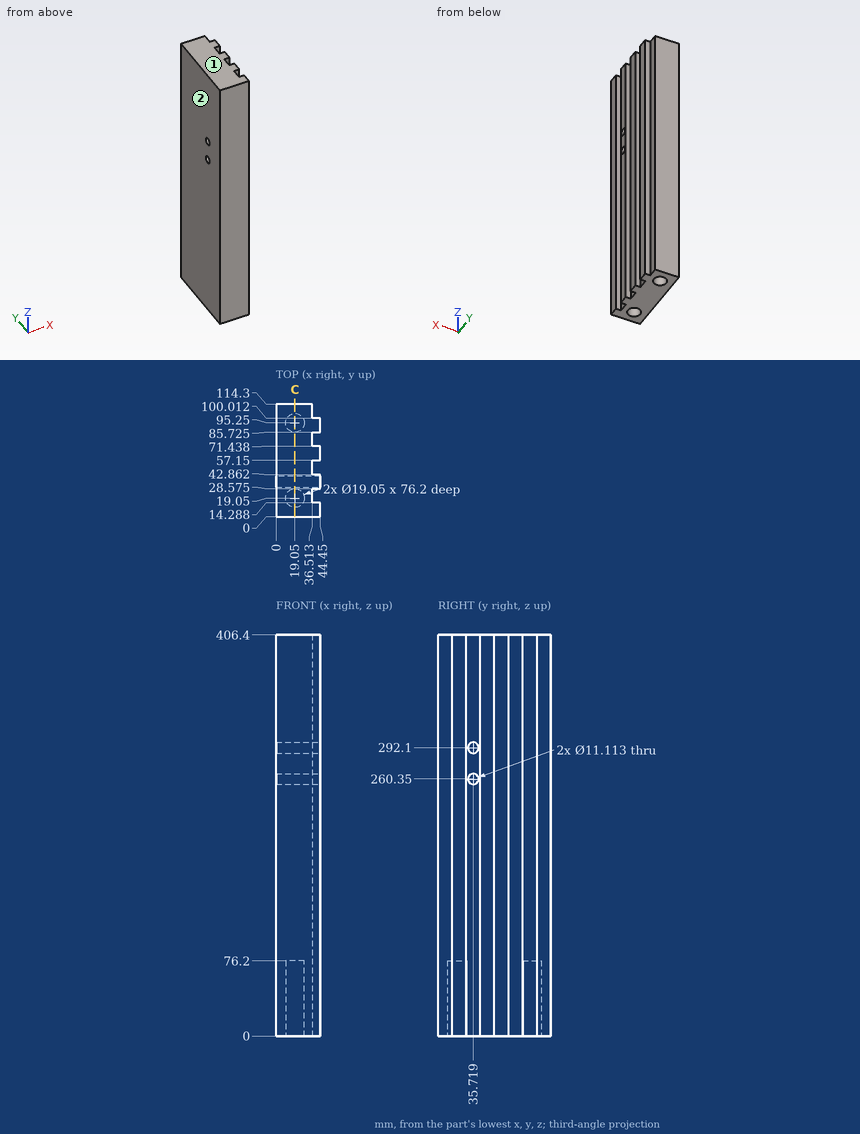
Here's the drawing with two shaded views (mm, measured from the low corner). I have some questions. Round coordinates to 2 decimals unless told otherwise and drop trailing zeros.
Item 1: If we mould it in two halves opening along X, with no side actions, what happens to the marked faces 1 and 2? For each: +X half, -X half, draft (parallel to the pull), parting line (faces both ways), or undercut.
Item 2: Suppose I cut it at C-C, the plane x = 19.05. State how many separate pieces and enclosed holes the cut face has, then the cut area to 3 significant figures.
Item 3: Will these pins go through, and if not, where does the flat tip stop? pin 1 Ø5.5 at (x, y) = (18, 97.5) entering from -Z; pin 2 Ø6 at (y, z) = (43.5, 94.5) entering from -X; pin 3 Ø7 at (y, z) = (18, 230.5) entering from +X; pin 4 Ø2.5 at (x, z) = (39.5, 171) entering from +Y.
Item 4: Please list where these lines run through material, in increasing order: L1, parallel to Y at x = 19.05, z = 42 (1 decimal); L2, parallel to X at y = 19, z = 16 (1 decimal); L3, parallel to Y at x = 16, z = 292 (1 decimal).
Reported:
1. face 1: draft
1. face 2: -X half
2. separate pieces: 1
2. enclosed holes: 2
2. area: 43,400 mm2
3. pin 1: stops at z = 76.2
3. pin 2: stops at x = 0
3. pin 3: stops at x = 36.51
3. pin 4: stops at y = 100.01
4. L1: y = 0 to 9.5, 28.6 to 85.7, 104.8 to 114.3
4. L2: x = 0 to 9.5, 28.6 to 36.5
4. L3: y = 0 to 30.2, 41.3 to 114.3
